from build123d import *

# Parameters (mm, degrees)
F0_R     = 10.5
F1_DEPTH = 4
F2_R     = 8
F3_DEPTH = 39
F7_DEPTH = 5


with BuildPart() as f1:
    # F0 (on Top) → F1 (new body)
    with BuildSketch(Plane.XY):
        Circle(F0_R)
    extrude(amount=F1_DEPTH)

    # F2 (on Top) → F3 (join)
    with BuildSketch(Plane.XY):
        Circle(F2_R)
    extrude(amount=F3_DEPTH)

    # F4 (on Right) → F5 (revolve)
    with BuildSketch(Plane.YZ):
        with BuildLine():
            Line((1, 43.898979), (0, 43.898979))
            Line((0, 43.898979), (0, 39))
            Line((0, 39), (5, 39))
            ThreePointArc((5, 39), (3.872983, 42.162278), (1, 43.898979))
        make_face()
    revolve(axis=Axis((0, 0, 41.5), (0, 0, -1)))

    # F6 (on face) → F7 (join)
    with BuildSketch(Plane.XY.offset(43.898979)):
        Polygon((0.441064, -0.897476), (0.997769, -0.066766), (0.556705, 0.83071), (-0.441064, 0.897476), (-0.997769, 0.066766), (-0.556705, -0.83071), align=None)
    extrude(amount=F7_DEPTH)


solid = f1.part
Geometry check sheet. Reference: the model listing, model coordinates, mm. A direction names the side the tool comes from. Round coordinates to 2 decimals unless told otherwise and drop trailing zeros. Write each loop counter-clockwise with the first axis right and the second up, starting at its lowest first coordinate (ties: lowest second). Pieces come first, ordered by that corner, then holes. Notation, with made-up numbers: (-37, 78) -> (5, 78) arc R10 cw to (5, 96) -> close; hole circle Ø2 at (65, 52.5). An arc over 180 degrees is marked (long way). One line per item, written item: value. Start each with the question number.
(1) Scan lines: line 1 (Z direction, x = -1.5, y = 9); line 2 (Z direction, x = -1.75, y = 6.5); line 3 (Y direction, x = 5.5, z = 30). Record each from-to range of solid material in increasing order. Write a range as [from, to].
(2) Cross-section at B-B, the plane x = 5.5. Record the cut outline in (y, z).
(3) Cross-section at D-D, the plane y = 9. Record the cut outline in (x, z).
(4) Go/stop test with flat-tipped pins: pin 1 Ø5 at (y, z) = (-0.5, 17) entering from -X; pin 2 Ø3 at (y, z) = (4, 5) entering from +X; pin 3 Ø1.5 at (y, z) = (-5.5, 21) entering from -X; pin 4 Ø2 at (x, y) = (-1.5, 0) entering from +Z. Record where each tip stops, or that it passes through.
(5) Cross-section at C-C, the plane z = 3. Record the cut outline in (x, y).
(6) Access from +Z, -Z, +X, -X, +Y, -Y to the whole of each face (thin tool, end or side, straight path). Record for faces 1 (the flat face through (5.2, 0.1, 39)), 2 (the flat face through (-0.065, -0.864, 46.364)), 3 (the flat face through (0.065, 0.864, 46.364)).
(7) Cross-section at A-A, the plane y = -6. Record the cut outline in (x, z).
Answer:
1. line 1: [0, 4]
1. line 2: [0, 39]
1. line 3: [-5.81, 5.81]
2. outline: (-8.94, 0) -> (8.94, 0) -> (8.94, 4) -> (5.81, 4) -> (5.81, 39) -> (-5.81, 39) -> (-5.81, 4) -> (-8.94, 4) -> close
3. outline: (-5.41, 0) -> (5.41, 0) -> (5.41, 4) -> (-5.41, 4) -> close
4. pin 1: x = -8
4. pin 2: x = 10.1
4. pin 3: x = -6.44
4. pin 4: z = 48.9
5. outline: circle Ø21 at (0, 0)
6. face 1: +Z
6. face 2: +Z, -X, -Y
6. face 3: +Z, +X, +Y
7. outline: (-8.62, 0) -> (8.62, 0) -> (8.62, 4) -> (5.29, 4) -> (5.29, 39) -> (-5.29, 39) -> (-5.29, 4) -> (-8.62, 4) -> close
